Design review of the part built by this model. Coordinates are the model's own, in mm. A direction names the side the tool comes from. Coordinates: 2 decimals unless noted, no trailing zeros. Loops run counter-clockwise (first coordinate to the right, second up) from the corner with the lowest first, then second, coordinate; pieces in that order, holes last. Notation, with made-up numbers: (68.25, -39.75) -> (90.25, -39.75) arc R29 ccw to (90.25, -0.75) -> close; hole circle Ø1 at (82, 47.25). An arc over 180 degrees is marked (long way). One line per item, written item: value. Start each with the question number.
1. Draft analysis for pull direction Z (two halves, no side actions). For faces 1 (the flat face through (2, 5, 34)), 2 (the flat face through (-3.9, 11, 43)), 3 (the flat face through (-12.6, 1.4, 1.2)), 4 (the flat face through (2, 2.5, 37)), state which applies: pulls with the +Z half, pulls with the -Z half, needs draft (parallel to the pull), parting line crosses it, or undercut.
2. Insertion check: pin 1 (9 mm diameter, centred on x = -1, z = 20, fed in from -Y); pin 2 (8 mm diameter, centred on x = -8.5, z = 21, fed in from +Y); pin 3 (10.5 mm diameter, centred on x = 1, z = 20.5, fed in from +Y); pin 4 (0.8 mm diameter, centred on y = 11, z = 43.5, fed in from +X). Each pin has a flat end and moves straight along its axis. Give the tip position at first contact, or say it passes through.
3. For probe 1 along Z at (x, y) = (-9.75, 4.5); probe 2 along Z at (x, y) = (0, 3.25); probe 3 along Z at (x, y) = (0, 6.1), list the stretches that pass through material, from the lowest coordinate up.
4. Add section A-A on x = 0. Write out the cut boundary in (y, z), plus the area to 3 significant figures.
5. Machinability: for faces 5 (the flat face through (3.9, 11, 43)), 6 (the cylindrical face through (-4.05, 2.17, 18.78)), 7 (the flat face through (1.8, 8, 33.5)), which of the approach directions +Z, -Z, +X, -X, +Y, -Y give a long, thin tool a straight path to every point of the face, cutting with its end or side? Answer none if there is none.
6. Add section B-B on z = 22.5. Write out the cut boundary in (x, y).
7. Add section D-D on y = 11. Write out the cut boundary in (x, z).
8. Add section C-C on y = 5.75. Write out the cut boundary in (x, z), plus the area to 3 significant figures.
```python
from build123d import *

# Parameters (mm, degrees)
CYLINDER001_R     = 5.5
CYLINDER001_DEPTH = 10
CYLINDER_R        = 2.15
CYLINDER_DEPTH    = 10
BOX001_W          = 29
BOX001_H          = 7.5
BOX001_DEPTH      = 35.5
BOX_W             = 29
BOX_H             = 10
BOX_DEPTH         = 45
CHAMFER_SIZE      = 2
BOX003_W          = 7.8
BOX003_H          = 3
BOX003_DEPTH      = 4.75
BOX002_W          = 27
BOX002_H          = 6
BOX002_DEPTH      = 23
CHAMFER001_SIZE   = 1
BOX004_W          = 7.8
BOX004_H          = 3
BOX004_DEPTH      = 4.75
CHAMFER002_SIZE   = 0.4
CHAMFER003_SIZE   = 0.4


with BuildPart() as cylinder001:
    # Cylinder001 → Cylinder001 (new body)
    with BuildSketch(Plane(origin=(0, -6, 22.5), x_dir=(1, 0, 0), z_dir=(0, 1, 0))):
        Circle(CYLINDER001_R)
    extrude(amount=CYLINDER001_DEPTH)


with BuildPart() as cylinder:
    # Cylinder → Cylinder (new body)
    with BuildSketch(Plane(origin=(0, 0, 22.5), x_dir=(1, 0, 0), z_dir=(0, 1, 0))):
        Circle(CYLINDER_R)
    extrude(amount=CYLINDER_DEPTH)


with BuildPart() as cube001:
    # Box001 → Box001 (new body)
    with BuildSketch(Plane(origin=(-11, 2.5, 4.75), x_dir=(1, 0, 0), z_dir=(0, 0, 1))):
        with Locations((14.5, 3.75)):
            Rectangle(BOX001_W, BOX001_H)
    extrude(amount=BOX001_DEPTH)


with BuildPart() as chamfer_body:
    # Box → Box (new body)
    with BuildSketch(Plane(origin=(-14, 0, 0), x_dir=(1, 0, 0), z_dir=(0, 0, 1))):
        with Locations((14.5, 5)):
            Rectangle(BOX_W, BOX_H)
    extrude(amount=BOX_DEPTH)

    # Cut: cut Cube001
    add(cube001.part, mode=Mode.SUBTRACT)

    # Chamfer
    chamfer_edges = [chamfer_body.edges().sort_by_distance(p)[0] for p in [
        (-14, 0, 22.5),
        (-14, 5, 45),
        (-14, 5, 0),
        (0.5, 0, 0),
        (0.5, 0, 45),
    ]]
    chamfer(chamfer_edges, length=CHAMFER_SIZE)


with BuildPart() as cube003:
    # Box003 → Box003 (new body)
    with BuildSketch(Plane(origin=(-3.9, 9, 0), x_dir=(1, 0, 0), z_dir=(0, 0, 1))):
        with Locations((3.9, 1.5)):
            Rectangle(BOX003_W, BOX003_H)
    extrude(amount=BOX003_DEPTH)


with BuildPart() as chamfer001:
    # Box002 → Box002 (new body)
    with BuildSketch(Plane(origin=(-12, 2.5, 11), x_dir=(1, 0, 0), z_dir=(0, 0, 1))):
        with Locations((13.5, 3)):
            Rectangle(BOX002_W, BOX002_H)
    extrude(amount=BOX002_DEPTH)

    # Chamfer001
    chamfer001_edges = [chamfer001.edges().sort_by_distance(p)[0] for p in [
        (1.5, 8.5, 11),
        (1.5, 8.5, 34),
    ]]
    chamfer(chamfer001_edges, length=CHAMFER001_SIZE)


with BuildPart() as chamfer003:
    # Box004 → Box004 (new body)
    with BuildSketch(Plane(origin=(-3.9, 9, 40.25), x_dir=(1, 0, 0), z_dir=(0, 0, 1))):
        with Locations((3.9, 1.5)):
            Rectangle(BOX004_W, BOX004_H)
    extrude(amount=BOX004_DEPTH)

    # Fusion: union Cube003, Chamfer001
    add(cube003.part)
    add(chamfer001.part)

    # Chamfer002
    chamfer002_edges = [chamfer003.edges().sort_by_distance(p)[0] for p in [
        (-3.9, 12, 42.625),
        (3.9, 12, 42.625),
        (-3.9, 12, 2.375),
        (3.9, 12, 2.375),
    ]]
    chamfer(chamfer002_edges, length=CHAMFER002_SIZE)

    # Fusion001: union Chamfer body
    add(chamfer_body.part)

    # Cut001: cut Cylinder
    add(cylinder.part, mode=Mode.SUBTRACT)

    # Cut002: cut Cylinder001
    add(cylinder001.part, mode=Mode.SUBTRACT)

    # Chamfer003
    chamfer003_edges = [chamfer003.edges().sort_by_distance(p)[0] for p in [
        (-5.5, 0, 22.5),
    ]]
    chamfer(chamfer003_edges, length=CHAMFER003_SIZE)


solid = chamfer003.part
```
Worked answers:
1. face 1: undercut
1. face 2: needs draft
1. face 3: pulls with the -Z half
1. face 4: undercut
2. pin 1: stops at y = 0
2. pin 2: stops at y = 10
2. pin 3: stops at y = 8.5
2. pin 4: stops at x = 3.9
3. probe 1: z = 0 to 4.75, 11 to 34, 40.25 to 45
3. probe 2: z = 0 to 4.75, 11 to 17, 28 to 34, 40.25 to 45
3. probe 3: z = 0 to 4.75, 11 to 20.35, 24.65 to 34, 40.25 to 45
4. outline: (0, 2) -> (2, 0) -> (12, 0) -> (12, 4.75) -> (2.5, 4.75) -> (2.5, 11) -> (7.5, 11) -> (8.5, 12) -> (8.5, 20.35) -> (4, 20.35) -> (4, 17) -> (0.4, 17) -> (0, 16.6) -> close; (0, 28.4) -> (0.4, 28) -> (4, 28) -> (4, 24.65) -> (8.5, 24.65) -> (8.5, 33) -> (7.5, 34) -> (2.5, 34) -> (2.5, 40.25) -> (12, 40.25) -> (12, 45) -> (2, 45) -> (0, 43) -> close
4. area: 272 mm²
5. face 5: +Z, -Z, +X, +Y
5. face 6: -Y
5. face 7: +X, +Y
6. outline: (-14, 2) -> (-12, 0) -> (-5.9, 0) -> (-5.5, 0.4) -> (-5.5, 4) -> (-2.15, 4) -> (-2.15, 8.5) -> (-11, 8.5) -> (-11, 10) -> (-14, 10) -> close; (2.15, 4) -> (5.5, 4) -> (5.5, 0.4) -> (5.9, 0) -> (15, 0) -> (15, 8.5) -> (2.15, 8.5) -> close
7. outline: (-3.9, 0) -> (3.9, 0) -> (3.9, 4.75) -> (-3.9, 4.75) -> close; (-3.9, 40.25) -> (3.9, 40.25) -> (3.9, 45) -> (-3.9, 45) -> close
8. outline: (-14, 2) -> (-12, 0) -> (15, 0) -> (15, 4.75) -> (-11, 4.75) -> (-11, 11) -> (15, 11) -> (15, 34) -> (-11, 34) -> (-11, 40.25) -> (15, 40.25) -> (15, 45) -> (-12, 45) -> (-14, 43) -> close; hole circle Ø4.3 at (0, 22.5)
8. area: 961 mm²
